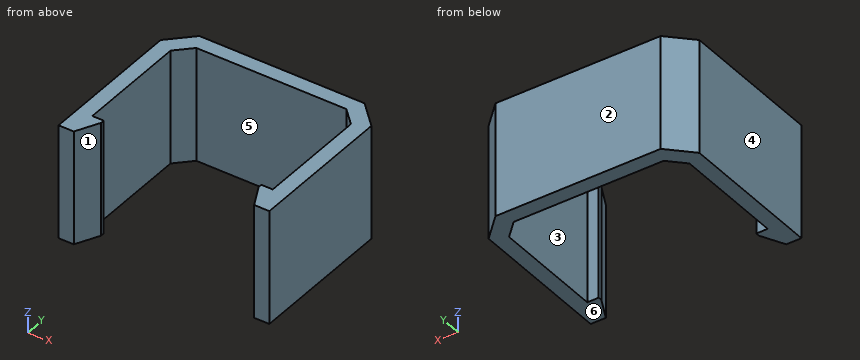
from build123d import *

# Parameters (mm, degrees)
BOSS_EXTRUDE1_DEPTH = 15
CHAMFER1_SIZE       = 3
CHAMFER2_SIZE       = 2
CHAMFER3_SIZE       = 1.5
CHAMFER3_SIZE2      = 3
CHAMFER4_SIZE       = 3
CHAMFER4_SIZE2      = 1.5


with BuildPart() as part:
    # Sketch1 → Boss-Extrude1 (new body)
    with BuildSketch(Plane.XY):
        Polygon((1.5, 0), (0, 0), (0, 16.75), (11.875, 16.75), (11.875, 18.75), (-2, 18.75), (-2, -3.5), (1.5, -3.5), align=None)
        Polygon((11.875, 18.75), (11.875, 16.75), (23.75, 16.75), (23.75, 0), (22.25, 0), (22.25, -3.5), (25.75, -3.5), (25.75, 18.75), align=None)
    extrude(amount=BOSS_EXTRUDE1_DEPTH)

    # Chamfer1
    chamfer1_edges = [part.edges().sort_by_distance(p)[0] for p in [
        (25.75, 18.75, 7.5),
        (-2, 18.75, 7.5),
    ]]
    chamfer(chamfer1_edges, length=CHAMFER1_SIZE)

    # Chamfer2
    chamfer2_edges = [part.edges().sort_by_distance(p)[0] for p in [
        (23.75, 16.75, 7.5),
        (0, 16.75, 7.5),
    ]]
    chamfer(chamfer2_edges, length=CHAMFER2_SIZE)

    # Chamfer3
    chamfer3_edges = [part.edges().sort_by_distance(p)[0] for p in [
        (1.5, -3.5, 7.5),
    ]]
    chamfer3_side = [part.faces().sort_by_distance(p)[0] for p in [
        (-0.25, -3.5, 7.5),
    ]]
    chamfer(chamfer3_edges, length=CHAMFER3_SIZE, length2=CHAMFER3_SIZE2, reference=chamfer3_side[0])

    # Chamfer4
    chamfer4_edges = [part.edges().sort_by_distance(p)[0] for p in [
        (22.25, -3.5, 7.5),
    ]]
    chamfer4_side = [part.faces().sort_by_distance(p)[0] for p in [
        (22.25, -1.75, 7.5),
    ]]
    chamfer(chamfer4_edges, length=CHAMFER4_SIZE, length2=CHAMFER4_SIZE2, reference=chamfer4_side[0])


solid = part.part
Read the model definition and answer for the solid it produces. Units are mm, in the model's axes. Face numbers are marked on the shaded views. A direction names the side the tool comes from. Round coordinates to 2 decimals unless told otherwise and drop trailing zeros. Write each loop counter-clockwise with the first axis right and the second up, starting at its lowest first coordinate (ties: lowest second). Pieces come first, ordered by that corner, then holes. Notation, with made-up numbers: M -18.5,71 L 16.5,71 A22 cw 16.5,87 Z; hole C -37.75,79 d2. An arc over 180 degrees is marked long. Use a Markdown table: item, result.
1) The part is cut by section A-A (y = -1.5). Write down the section's boundary in (x, z), plus the area to 3 significant figures.
Answers follow:
| item | result |
|---|---|
| outline | M -2,0 L 1,0 L 1,15 L -2,15 Z; M 22.75,0 L 25.75,0 L 25.75,15 L 22.75,15 Z |
| area | 90.0 mm2 |
2) A flat-ended cylindrical pin translates along its axis: pin 1 (1 mm diameter, centred on x = 15, z = 6.5, fed in from -Y). Find the tip coordinate at first contact, or state that the pin passes through.
Answers follow:
| item | result |
|---|---|
| pin 1 | stops at y = 16.75 |
3) The part is cut by section B-B (z = 1.75). Write down the section's boundary in (x, y).
Answers follow:
| item | result |
|---|---|
| outline | M -2,-3.5 L 0,-3.5 L 1.5,-0.5 L 1.5,0 L 0,0 L 0,14.75 L 2,16.75 L 21.75,16.75 L 23.75,14.75 L 23.75,0 L 22.25,0 L 22.25,-0.5 L 23.75,-3.5 L 25.75,-3.5 L 25.75,15.75 L 22.75,18.75 L 1,18.75 L -2,15.75 Z |
4) The part is cut by section D-D (y = 17.25). Write down the section's boundary in (x, z).
Answers follow:
| item | result |
|---|---|
| outline | M -0.5,0 L 24.25,0 L 24.25,15 L -0.5,15 Z |
5) For a pull along X with two mould halves and no side action, classify the marked faces 4, 5 and 6 as pulls with the +X half, pulls with the -X half, needs draft (parallel to the pull), parting line crosses it, or undercut.
Answers follow:
| item | result |
|---|---|
| face 4 | pulls with the -X half |
| face 5 | undercut |
| face 6 | needs draft |
6) Straight lines are drawn through the part: line 1 along X through (y, z) = (4.75, 11.5); line 2 along Y through (x, z) = (4.5, 11.5); line 3 along Y through (x, z) = (1, 13.5). For each, find the intervals that lie inside material, in ascending order. Write a range as [from, to].
Answers follow:
| item | result |
|---|---|
| line 1 | x = [-2, 0], [23.75, 25.75] |
| line 2 | y = [16.75, 18.75] |
| line 3 | y = [-1.5, 0], [15.75, 18.75] |
7) The part is cut by section C-C (y = 13). Write down the section's boundary in (x, z), plus the area to 3 significant figures.
Answers follow:
| item | result |
|---|---|
| outline | M -2,0 L 0,0 L 0,15 L -2,15 Z; M 23.75,0 L 25.75,0 L 25.75,15 L 23.75,15 Z |
| area | 60.0 mm2 |
8) A tool of negligible diameter and unlimited length cuts with its end or side. For the marked faces 1, 2 and 3, from which of +Z, -Z, +X, -X, +Y, -Y can it reach the whole face along a straight path? Write none if from no direction.
Answers follow:
| item | result |
|---|---|
| face 1 | +Z, -Z, -Y |
| face 2 | +Z, -Z, +X, -X, +Y |
| face 3 | +Z, -Z |
